from build123d import *

# Parameters (mm, degrees)
F1_DEPTH = 60
F2_R     = 9.656854
F3_R     = 16.014444
F4_DEPTH = 101


with BuildPart() as f1:
    # F0 (on Front) → F1 (new body)
    with BuildSketch(Plane.XZ):
        Polygon((18.220022, 60.063125), (-58.951251, 60.063125), (-58.951251, -46.7043), (-27.914977, -46.7043), (-27.914977, -13.151571), (17.381208, -13.151571), (17.381208, -46.7043), (48.417483, -46.7043), (48.417483, 18.961032), (18.220022, 18.961032), align=None)
    extrude(amount=F1_DEPTH)

    # F2
    f2_edges = [f1.edges().sort_by_distance(p)[0] for p in [
        (18.220022, -30, 60.063125),
        (48.417483, -30, 18.961032),
    ]]
    fillet(f2_edges, radius=F2_R)

    # F3 (on face) → F4 (cut)
    with BuildSketch(Plane.XZ.offset(60)):
        with Locations((-23.123993, 25.327024)):
            Circle(F3_R)
    extrude(amount=-F4_DEPTH, mode=Mode.SUBTRACT)


solid = f1.part
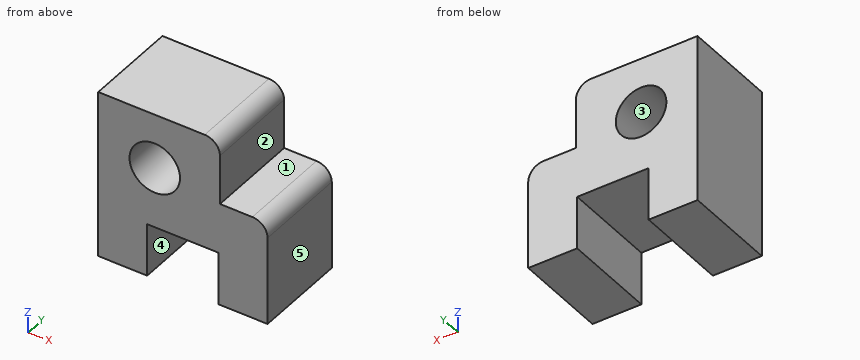
Input: part model. Units: mm. Frame: model coordinates. Face numbers are marked on the shaded views. A direction names the side the tool comes from. Round coordinates to 2 decimals unless told otherwise and drop trailing zeros. Order: outer loops, then holes, each group sorted by start corner. A loop starts at its lowest first (then second) coordinate and runs counter-clockwise, first axis right, second up. Notation, with made-up numbers: (6, 85) - (45, 85) arc R33 cw to (45, 119) - close; hole circle Ø7 at (8, 24). An arc over 180 degrees is marked (long way). Answer as a JSON object with one key per item and string values. Group by question number.
(1) Cut plane D-D (x = 28). Return loops of the section in (y, z), then the cut area to 3 significant figures.
(2) Material intervals for probe 1 along X at (y, z) = (-15.5, -38.5); probe 2 along X at (y, z) = (-3.5, 44.5); probe 3 along Z at (x, y) = (35, -15), sorted ascending. Write a range as from..to.
(3) Draft query along X for the marked faces 1, 2 and 3. Return one class per face: released by +X, released by -X, zero draft, split by the parting line, or undercut.
(4) Reachability of the marked faces 4 and 5 from +Z, -Z, +X, -X, +Y, -Y: full face, straight path, thin tool, end or side. Return the list, or none.
(5) Pin query (flat end, axial travel): P1, Ø9.5, axis at y = -42.5, z = 35.5, coming from the +X side; P2, Ø5, axis at x = 14, y = -50, coming from the -Z side; P3, Ø16.5, axis at x = 25, y = -39.5, coming from the +Z side. Return the tip coordinate at first contact, or that it passes through.
(6) Cut plane B-B (x = -15). Return loops of the section in (y, z), then the cut area to 3 significant figures.
(7) Cut plane A-A (z = -20). Return loops of the section in (x, y), then the cut area to 3 significant figures.
(8) Cut plane C-C (y = -53). Return loops of the section in (x, z).
Here are the results:
{
 "1": {"outline": "(-60, -46.7) - (0, -46.7) - (0, 18.96) - (-60, 18.96) - close", "area": "3,940 mm^2"},
 "2": {"probe 1": "x = -58.95..-27.91, 17.38..48.42", "probe 2": "x = -58.95..18.22", "probe 3": "z = -46.7..18.96"},
 "3": {"face 1": "zero draft", "face 2": "released by +X", "face 3": "undercut"},
 "4": {"face 4": "-Z, +Y, -Y", "face 5": "+Z, -Z, +X, +Y, -Y"},
 "5": {"P1": "stops at x = 18.22", "P2": "stops at z = -13.15", "P3": "stops at z = 55.53"},
 "6": {"outline": "(-60, -13.15) - (0, -13.15) - (0, 11.53) - (-60, 11.53) - close; (-60, 39.13) - (0, 39.13) - (0, 60.06) - (-60, 60.06) - close", "area": "2,740 mm^2"},
 "7": {"outline": "(-58.95, -60) - (-27.91, -60) - (-27.91, 0) - (-58.95, 0) - close; (17.38, -60) - (48.42, -60) - (48.42, 0) - (17.38, 0) - close", "area": "3,720 mm^2"},
 "8": {"outline": "(-58.95, -46.7) - (-27.91, -46.7) - (-27.91, -13.15) - (17.38, -13.15) - (17.38, -46.7) - (48.42, -46.7) - (48.42, 9.3) arc R9.66 ccw to (38.76, 18.96) - (18.22, 18.96) - (18.22, 50.41) arc R9.66 ccw to (8.56, 60.06) - (-58.95, 60.06) - close; hole circle Ø32.03 at (-23.12, 25.33)"}
}
